For this review, take the finished solid that the model builds, in its own axes (mm). A direction names the side the tool comes from. Round coordinates to 2 decimals unless told otherwise and drop trailing zeros. Write each loop counter-clockwise with the first axis right and the second up, starting at its lowest first coordinate (ties: lowest second). Pieces come first, ordered by that corner, then holes. Notation, with made-up numbers: (-3.75, 52) -> (38.25, 52) arc R29 cw to (38.25, 86) -> close; hole circle Ø7 at (-27.5, 48.25). An arc over 180 degrees is marked (long way). Answer in a Markdown table with one row per item.
from build123d import *

# Parameters (mm, degrees)
SKETCH1_W                      = 96
SKETCH1_H                      = 121.5
SKETCH1_W_2                    = 86
SKETCH1_H_2                    = 98.5
BOSS_EXTRUDE1_DEPTH            = 2
SKETCH2_W                      = 100
SKETCH2_H                      = 125.5
SKETCH2_W_2                    = 96
SKETCH2_H_2                    = 121.5
BOSS_EXTRUDE2_DEPTH            = 5.2
CUT_EXTRUDE1_REACH             = 82.403
SKETCH3_R                      = 2.25
SKETCH3_R_2                    = 1.65
CUT_EXTRUDE1_DIRECTION_2_DEPTH = 81.402751819
FILLET1_R                      = 1.65
SKETCH4_W                      = 100
SKETCH4_H                      = 5.5
BOSS_EXTRUDE3_DEPTH            = 2
BOSS_EXTRUDE5_DEPTH            = 15


with BuildPart() as part:
    # Sketch1 → Boss-Extrude1 (new body)
    with BuildSketch(Plane(origin=(0, 0, 0), x_dir=(1, 0, 0), z_dir=(0, 1, 0))):
        Rectangle(SKETCH1_W, SKETCH1_H)
        with Locations((0, 6.5)):
            Rectangle(SKETCH1_W_2, SKETCH1_H_2, mode=Mode.SUBTRACT)
    extrude(amount=BOSS_EXTRUDE1_DEPTH)

    # Sketch2 → Boss-Extrude2 (add)
    with BuildSketch(Plane(origin=(0, 0, 0), x_dir=(1, 0, 0), z_dir=(0, 1, 0))):
        Rectangle(SKETCH2_W, SKETCH2_H)
        Rectangle(SKETCH2_W_2, SKETCH2_H_2, mode=Mode.SUBTRACT)
    extrude(amount=BOSS_EXTRUDE2_DEPTH)

    # Sketch3 → Cut-Extrude1 (cut, up to next)
    with BuildSketch(Plane.XZ, mode=Mode.PRIVATE) as cut_extrude1_sk1:
        with Locations(Location((25, 52.75, 0), (0, 0, 90))):
            Circle(SKETCH3_R)
    cut_extrude1_tool1 = extrude(cut_extrude1_sk1.sketch, amount=-CUT_EXTRUDE1_REACH, mode=Mode.PRIVATE) & part.part
    # Sketch3 → Cut-Extrude1 (cut, up to next)
    with BuildSketch(Plane.XZ, mode=Mode.PRIVATE) as cut_extrude1_sk2:
        with Locations(Location((-25, 52.75, 0), (0, 0, 90))):
            Circle(SKETCH3_R)
    cut_extrude1_tool2 = extrude(cut_extrude1_sk2.sketch, amount=-CUT_EXTRUDE1_REACH, mode=Mode.PRIVATE) & part.part
    # Sketch3 → Cut-Extrude1 (cut, up to next)
    with BuildSketch(Plane.XZ, mode=Mode.PRIVATE) as cut_extrude1_sk3:
        with Locations(Location((46.5, -59.25, 0), (0, 0, 24.619977329))):
            Circle(SKETCH3_R_2)
    cut_extrude1_tool3 = extrude(cut_extrude1_sk3.sketch, amount=-CUT_EXTRUDE1_REACH, mode=Mode.PRIVATE) & part.part
    # Sketch3 → Cut-Extrude1 (cut, up to next)
    with BuildSketch(Plane.XZ, mode=Mode.PRIVATE) as cut_extrude1_sk4:
        with Locations(Location((-46.5, -59.25, 0), (0, 0, 155.380022671))):
            Circle(SKETCH3_R_2)
    cut_extrude1_tool4 = extrude(cut_extrude1_sk4.sketch, amount=-CUT_EXTRUDE1_REACH, mode=Mode.PRIVATE) & part.part
    add(cut_extrude1_tool1.solids().sort_by_distance((25, 0, 52.75))[0], mode=Mode.SUBTRACT)
    add(cut_extrude1_tool2.solids().sort_by_distance((-25, 0, 52.75))[0], mode=Mode.SUBTRACT)
    add(cut_extrude1_tool3.solids().sort_by_distance((46.5, 0, -59.25))[0], mode=Mode.SUBTRACT)
    add(cut_extrude1_tool4.solids().sort_by_distance((-46.5, 0, -59.25))[0], mode=Mode.SUBTRACT)

    # Sketch3 → Cut-Extrude1 direction 2 (cut)
    with BuildSketch(Plane.XZ):
        with Locations(Location((25, 52.75, 0), (0, 0, 90))):
            Circle(SKETCH3_R)
        with Locations(Location((-25, 52.75, 0), (0, 0, 90))):
            Circle(SKETCH3_R)
        with Locations(Location((46.5, -59.25, 0), (0, 0, 24.619977329))):
            Circle(SKETCH3_R_2)
        with Locations(Location((-46.5, -59.25, 0), (0, 0, 155.380022671))):
            Circle(SKETCH3_R_2)
    extrude(amount=CUT_EXTRUDE1_DIRECTION_2_DEPTH, mode=Mode.SUBTRACT)

    # Fillet1
    # the kernel refuses this fillet: 1.65 mm, written as the material it adds along each edge
    with BuildSketch(Plane(origin=(48, 2, -60.75), x_dir=(0, 0, 1), z_dir=(0, 1, 0))) as fillet1_piece_1_section:
        with BuildLine():
            CenterArc((FILLET1_R, -FILLET1_R), FILLET1_R, 90, 90)
            Line((0, -FILLET1_R), (0, 0))
            Line((0, 0), (FILLET1_R, 0))
        make_face()
    fillet1_piece_1 = extrude(amount=3.2, mode=Mode.PRIVATE)
    fillet1_piece_1 = fillet1_piece_1 - Plane(origin=(46.5, 3.6, -59.25), x_dir=(0.9090909090884159, 0, 0.4165977904559716), z_dir=(0, -1, 0)) * Cylinder(1.65, 13, mode=Mode.PRIVATE)
    add(fillet1_piece_1)
    with BuildSketch(Plane(origin=(-48, 2, -60.75), x_dir=(1, 0, 0), z_dir=(0, 1, 0))) as fillet1_piece_2_section:
        with BuildLine():
            CenterArc((FILLET1_R, -FILLET1_R), FILLET1_R, 90, 90)
            Line((0, -FILLET1_R), (0, 0))
            Line((0, 0), (FILLET1_R, 0))
        make_face()
    fillet1_piece_2 = extrude(amount=3.2, mode=Mode.PRIVATE)
    fillet1_piece_2 = fillet1_piece_2 - Plane(origin=(-46.5, 3.6, -59.25), x_dir=(-0.9090909090884159, 0, 0.4165977904559715), z_dir=(0, -1, 0)) * Cylinder(1.65, 14, mode=Mode.PRIVATE)
    add(fillet1_piece_2)

    # Sketch4 → Boss-Extrude3 (add)
    with BuildSketch(Plane(origin=(0, 0, 0), x_dir=(1, 0, 0), z_dir=(0, 1, 0))):
        with Locations((0, 65.5)):
            Rectangle(SKETCH4_W, SKETCH4_H)
    extrude(amount=BOSS_EXTRUDE3_DEPTH)

    # Sketch7 → Boss-Extrude5 (add)
    with BuildSketch(Plane(origin=(0, 2, 0), x_dir=(1, 0, 0), z_dir=(0, 1, 0))):
        Polygon((-50, 68.25), (50, 68.25), (50, 62.75), (48, 62.75), (48, 66.25), (-50, 66.25), align=None)
    extrude(amount=BOSS_EXTRUDE5_DEPTH)


solid = part.part
1) Mouldability with a two-part tool opening along X and no side actions: class faces 1 (the flat face through (50, 3, -8)), 2 (the flat face through (-1, 3, 62.75)), 3 (the cylindrical face through (47.802, 1.986, -60.264)) as pulls with the +X half, pulls with the -X half, needs draft (parallel to the pull), parting line crosses it, or undercut.
Solved:
| item | result |
|---|---|
| face 1 | pulls with the +X half |
| face 2 | needs draft |
| face 3 | undercut |
2) Consider section D-D on y = 3.5. State the section outline as (x, z) points.
Solved:
| item | result |
|---|---|
| outline | (-50, -68.25) -> (50, -68.25) -> (50, 62.75) -> (-50, 62.75) -> (-50, -62.75) -> (48, -62.75) -> (48, -66.25) -> (-50, -66.25) -> close; hole (-48, -58.56) arc R1.65 ccw to (-45.81, -60.75) -> (45.81, -60.75) arc R1.65 ccw to (48, -58.56) -> (48, 60.75) -> (-48, 60.75) -> close |
3) Consider section C-C on x = 9. State the section outline as (y, z) points.
Solved:
| item | result |
|---|---|
| outline | (0, -68.25) -> (17, -68.25) -> (17, -66.25) -> (2, -66.25) -> (2, -62.75) -> (5.2, -62.75) -> (5.2, -60.75) -> (2, -60.75) -> (2, -55.75) -> (0, -55.75) -> close; (0, 42.75) -> (2, 42.75) -> (2, 60.75) -> (5.2, 60.75) -> (5.2, 62.75) -> (0, 62.75) -> close |
4) Consider section B-B on z = -48. State the section outline as (x, y) points.
Solved:
| item | result |
|---|---|
| outline | (-50, 0) -> (-43, 0) -> (-43, 2) -> (-48, 2) -> (-48, 5.2) -> (-50, 5.2) -> close; (43, 0) -> (50, 0) -> (50, 5.2) -> (48, 5.2) -> (48, 2) -> (43, 2) -> close |
5) For line 1 (Z direction, x = 25, y = 1); line 2 (X direction, y = 1, z = 52.75); line 3 (X direction, y = 1.9, z = -59.25), list the stretches that pass through material, from the lowest coordinate up. Write a range as [from, to].
Solved:
| item | result |
|---|---|
| line 1 | [-68.25, -55.75], [42.75, 50.5], [55, 62.75] |
| line 2 | [-50, -27.25], [-22.75, 22.75], [27.25, 50] |
| line 3 | [-50, -48.15], [-44.85, 44.85], [48.15, 50] |
6) For faces 4 (the flat face through (48, 4, 2)), 5 (the flat face through (0, 9, -66.25)), 6 (the cylindrical face through (-47.886, 1.986, -60.145)), 7 (the flat face through (48.4, 5.2, -0.3)), list the 3-axis set-ups (+Z, -Z, +X, -X, +Y, -Y) from which the entire face can be reached by the end or side of a thin tool; tool diameter is ignored.
Solved:
| item | result |
|---|---|
| face 4 | +Y |
| face 5 | -X, +Y |
| face 6 | +Y, -Y |
| face 7 | +Z, +X, -X, +Y |
7) Clearance check with flat-ended pins moving along their axes: pin 1 Ø5 at (x, z) = (-25, 52.75) entering from +Y; pin 2 Ø1 at (y, z) = (7, -52) entering from +X; pin 3 Ø0.6 at (x, y) = (49, 9.5) entering from +Z. State where each tip first meets the part, or that it passes through.
Solved:
| item | result |
|---|---|
| pin 1 | y = 2 |
| pin 2 | through |
| pin 3 | z = -62.75 |
8) Consider section A-A on x = -25. State the section outline as (y, z) points, then the cut area to 3 significant figures.
Solved:
| item | result |
|---|---|
| outline | (0, -68.25) -> (17, -68.25) -> (17, -66.25) -> (2, -66.25) -> (2, -62.75) -> (5.2, -62.75) -> (5.2, -60.75) -> (2, -60.75) -> (2, -55.75) -> (0, -55.75) -> close; (0, 42.75) -> (2, 42.75) -> (2, 50.5) -> (0, 50.5) -> close; (0, 55) -> (2, 55) -> (2, 60.75) -> (5.2, 60.75) -> (5.2, 62.75) -> (0, 62.75) -> close |
| area | 98.8 mm² |
